```python
from build123d import *

# Parameters (mm, degrees)
SKETCH_1_R          = 1.65
EXTRUDE_1_DEPTH     = 2.5
SKETCH_1_3_W        = 10
SKETCH_1_3_H        = 10
EXTRUDE_2_DEPTH     = 5
EXTRUDE_3_DEPTH     = 10
OTHER_START         = -2.194885141
OTHER_1_DEPTH       = 4.4
OTHER_START_2       = -4.194885141
OTHER_1_2_OUTLINE_R = 1.2
OTHER_1_2_DEPTH     = 7.198493548
CUT_EXTRUDE_START   = -9.201507
CUT_EXTRUDE_1_DEPTH = 4.400001


# Read off the part's stored shape, not the designer's step: Отступ1
with BuildPart() as part:
    # Эскиз1 → Бобышка-Вытянуть1 (new body)
    with BuildSketch(Plane.XY):
        Polygon((-4.846391593, 58.406906995), (-4.846391593, 55.11601046), (-1.996391593, 53.470562193), (0.853608407, 55.11601046), (0.853608407, 58.406906995), (-1.996391593, 60.052355262), align=None)
        with Locations((-1.996391593, 56.761458727)):
            Circle(SKETCH_1_R, mode=Mode.SUBTRACT)
    extrude(amount=EXTRUDE_1_DEPTH)

    # Эскиз1<3> → Бобышка-Вытянуть2 (add)
    with BuildSketch(Plane.XY):
        with Locations((-1.996391593, 56.761458727)):
            Rectangle(SKETCH_1_3_W, SKETCH_1_3_H)
        Polygon((-4.846391593, 55.11601046), (-1.996391593, 53.470562193), (0.853608407, 55.11601046), (0.853608407, 58.406906995), (-1.996391593, 60.052355262), (-4.846391593, 58.406906995), align=None, mode=Mode.SUBTRACT)
    extrude(amount=EXTRUDE_2_DEPTH)

    # Эскиз2 → Бобышка-Вытянуть3 (add)
    with BuildSketch(Plane(origin=(3.003608407, 0, 0), x_dir=(0, 0, -1), z_dir=(1, 0, 0))):
        with BuildLine():
            Line((0, 63.079006264), (0, 61.761458727))
            Line((0, 61.761458727), (-5, 61.761458727))
            Line((-5, 61.761458727), (-5, 63.079006264))
            ThreePointArc((-5, 63.079006264), (-2.5, 65.579006264), (0, 63.079006264))
        make_face()
    extrude(amount=-EXTRUDE_3_DEPTH)

    # Отступ1 outline → Отступ1 (cut)
    with BuildSketch(Plane.YZ.offset(OTHER_START)):
        with BuildLine():
            Line((65.153996838, 3.894422503), (63.084523903, 3.899992575))
            ThreePointArc((63.084523903, 3.899992575), (61.080242494, 2.30545954), (62.195830177, 0))
            Line((62.195830177, 0), (63.079006264, 0))
            ThreePointArc((63.079006264, 0), (65.285367098, 1.324427003), (65.153996838, 3.894422503))
        make_face()
    extrude(amount=OTHER_1_DEPTH, mode=Mode.SUBTRACT)

    # Other 1 2 outline → Other 1 2 (cut)
    with BuildSketch(Plane.YZ.offset(OTHER_START_2)):
        with Locations((63.079006264, 1.85)):
            Circle(OTHER_1_2_OUTLINE_R)
    extrude(amount=OTHER_1_2_DEPTH, mode=Mode.SUBTRACT)

    # Эскиз3 → Вырез-Вытянуть1 (cut)
    with BuildSketch(Plane.ZY.offset(6.996391593).offset(CUT_EXTRUDE_START)):
        with BuildLine():
            ThreePointArc((0, 58.061458727), (2.5, 60.561458727), (5, 58.061458727))
            Line((5, 58.061458727), (5, 63.079006264))
            ThreePointArc((5, 63.079006264), (2.5, 65.579006264), (0, 63.079006264))
            Line((0, 63.079006264), (0, 58.061458727))
        make_face()
    extrude(amount=CUT_EXTRUDE_1_DEPTH, mode=Mode.SUBTRACT)


solid = part.part
```
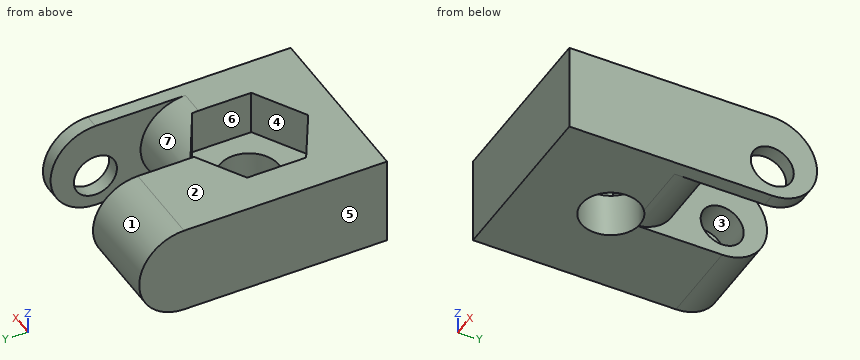
Geometry: final body of the model. Coordinates: model frame, mm. Face numbers are marked on the shaded views. A direction names the side the tool comes from. Round coordinates to 2 decimals unless told otherwise and drop trailing zeros. Loops run counter-clockwise (first coordinate to the right, second up) from the corner with the lowest first, then second, coordinate; pieces in that order, holes last. Notation, with made-up numbers: (12.5, 72) -> (44.5, 72) arc R16 cw to (44.5, 82) -> close; hole circle Ø11 at (0.5, -20.75). An arc over 180 degrees is marked (long way). Use one line per item in the form item = value.
Item 1: Access query for the marked faces 5, 6 and 7. Directions: +Z, -Z, +X, -X, +Y, -Y. A direction counts if a zero-diameter tool reaches every point of the face in a straight line with its end or side. Return the directions, or none.
Evaluation:
face_5 = +Z, -Z, -X, +Y, -Y
face_6 = +Z
face_7 = +Y
Item 2: Cut plane B-B on x = -3. Output: boundary loops of the cut face in (y, z), then the cut area to 3 significant figures.
Evaluation:
outline = (51.76, 0) -> (55.45, 0) -> (55.45, 2.5) -> (54.05, 2.5) -> (54.05, 5) -> (51.76, 5) -> close; (58.07, 0) -> (63.08, 0) arc R2.5 ccw to (63.08, 5) -> (59.47, 5) -> (59.47, 2.5) -> (58.07, 2.5) -> close; hole circle Ø2.4 at (63.08, 1.85)
area = 41.8 mm2
Item 3: Contact query for flat-ended pins moving along their axis: pin 1 Ø2 at (x, y) = (-0.5, 60.5) entering from -Z; pin 2 Ø0.7 at (y, z) = (63, 2) entering from +X; pin 3 Ø4.5 at (x, y) = (-2, 56.76) entering from +Z. Output: stop coordinate, or through.
Evaluation:
pin_1 = 0.46
pin_2 = -4.19
pin_3 = 2.5
Item 4: Cut plane A-A on z = 1.85. Output: boundary loops of the cut face in (x, y).
Evaluation:
outline = (-7, 51.76) -> (3, 51.76) -> (3, 61.88) -> (2.21, 61.88) -> (2.21, 60.48) -> (-2.19, 60.48) -> (-2.19, 61.88) -> (-4.19, 61.88) -> (-4.19, 64.28) -> (-2.19, 64.28) -> (-2.19, 65.49) -> (-7, 65.49) -> close; (2.21, 64.28) -> (3, 64.28) -> (3, 65.49) -> (2.21, 65.49) -> close; hole circle Ø3.3 at (-2, 56.76)
Item 5: Cut plane C-C on y = 55.5. Output: boundary loops of the cut face in (x, z), then the cut area to 3 significant figures.
Evaluation:
outline = (-7, 0) -> (-3.06, 0) -> (-3.06, 2.5) -> (-4.85, 2.5) -> (-4.85, 5) -> (-7, 5) -> close; (-0.93, 0) -> (3, 0) -> (3, 5) -> (0.85, 5) -> (0.85, 2.5) -> (-0.93, 2.5) -> close
area = 30.4 mm2
Item 6: Draft query along Z for the marked faces 1, 2, 3 and 4. Return one class per face: released by +Z, released by -Z, zero draft, split by the parting line, or undercut.
Evaluation:
face_1 = split by the parting line
face_2 = released by +Z
face_3 = undercut
face_4 = zero draft
Item 7: Material intervals for probe 1 along X at (y, z) = (63.5, 4.1); probe 2 along Y at (x, z) = (-3.25, 1.85); probe 3 along X at (y, z) = (57, 2.45), sorted ascending.
Evaluation:
probe_1 = -7 to -2.19, 2.21 to 3
probe_2 = 51.76 to 55.69, 57.83 to 61.88, 64.28 to 65.49
probe_3 = -7 to -3.63, -0.36 to 3
Item 8: Cut plane D-D on y = 62.5. Output: boundary loops of the cut face in (x, z), then the cut area to 3 significant figures.
Evaluation:
outline = (-7, 0) -> (-2.19, 0) -> (-2.19, 0.8) -> (-4.19, 0.8) -> (-4.19, 2.9) -> (-2.19, 2.9) -> (-2.19, 5) -> (-7, 5) -> close; (2.21, 0) -> (3, 0) -> (3, 0.8) -> (2.21, 0.8) -> close; (2.21, 2.9) -> (3, 2.9) -> (3, 5) -> (2.21, 5) -> close
area = 22.1 mm2
